The model under review builds one solid part; all positions refer to its coordinate system, in mm. Face numbers are marked on the shaded views. A direction names the side the tool comes from. Coordinates: 2 decimals unless noted, no trailing zeros. Loops run counter-clockwise (first coordinate to the right, second up) from the corner with the lowest first, then second, coordinate; pieces in that order, holes last. Notation, with made-up numbers: M 41,25 L 78,25 A12 cw 78,43 Z; hole C 9,25.25 d9. An arc over 180 degrees is marked long. Use one line per item in the form item = value.
```python
from build123d import *

# Parameters (mm, degrees)
DODANIE_WYCI_GNI_CIE1_DEPTH       = 25
DODANIE_WYCI_GNI_CIE2_DEPTH       = 5
WYCI_GNI_CIE_CIENKA_CIANKA1_DEPTH = 70
ZAOKR_GLENIE1_R                   = 10


with BuildPart() as part:
    # Szkic1 → Dodanie-wyci_gni_cie1 (new body)
    with BuildSketch(Plane.XY):
        with BuildLine():
            Line((0, 15), (0, 20))
            ThreePointArc((0, 20), (-20, 0), (0, -20))
            Line((0, -20), (0, -15))
            ThreePointArc((0, -15), (-15, 0), (0, 15))
        make_face()
    extrude(amount=DODANIE_WYCI_GNI_CIE1_DEPTH)

    # Szkic2 → Dodanie-wyci_gni_cie2 (add)
    with BuildSketch(Plane.XY):
        with BuildLine():
            Line((0, 20), (0, 72))
            Line((0, 72), (-40, 72))
            Line((-40, 72), (-40, 50.70936694))
            ThreePointArc((-40, 50.70936694), (-58.888387013, -17.302808514), (0, -56.220478651))
            Line((0, -56.220478651), (0, -20))
            Line((0, -20), (0, -15))
            ThreePointArc((0, -15), (-15, 0), (0, 15))
            Line((0, 15), (0, 20))
        make_face()
    extrude(amount=DODANIE_WYCI_GNI_CIE2_DEPTH)


with BuildPart() as body_2:
    # Lustro4: mirrored copy
    add(part.part.mirror(Plane(origin=(0, 0, -35), x_dir=(1, 0, 0), z_dir=(0, 0, -1))))


with BuildPart() as part_1:
    add(part.part)

    add(body_2.part)  # Wyci_gni_cie-cienka _cianka1 merges body 2
    # Szkic14 → Wyci_gni_cie-cienka _cianka1 (add)
    with BuildSketch(Plane(origin=(0, 0, 0), x_dir=(-1, 0, 0), z_dir=(0, 0, -1))):
        with BuildLine():
            Line((40, 72), (40, 50.70936694))
            ThreePointArc((40, 50.70936694), (58.888387013, -17.302808514), (0, -56.220478651))
            Line((0, -56.220478651), (0.224300204, -51.225512243))
            ThreePointArc((0.224300204, -51.225512243), (54.609267077, -14.434561812), (35, 48.229425454))
            Line((35, 48.229425454), (35, 72))
            Line((35, 72), (40, 72))
        make_face()
    extrude(amount=WYCI_GNI_CIE_CIENKA_CIANKA1_DEPTH)

    # Zaokr_glenie1
    zaokr_glenie1_edges = [part_1.edges().sort_by_distance(p)[0] for p in [
        (-40, 61.35468347, 5),
        (-40, 61.35468347, -75),
    ]]
    fillet(zaokr_glenie1_edges, radius=ZAOKR_GLENIE1_R)


solid = part_1.part
```
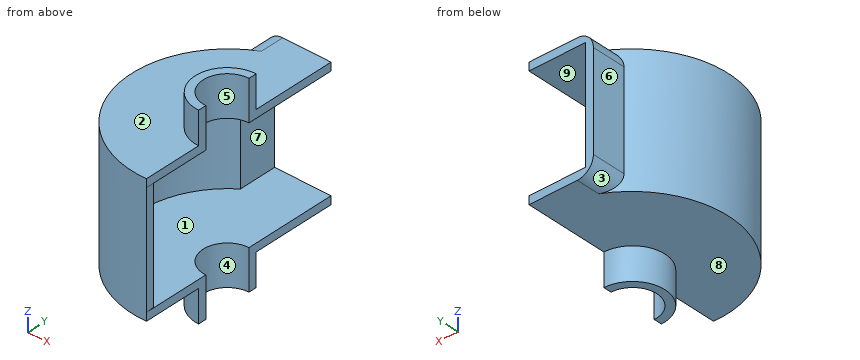
1. The part is to be moulded in two halves that separate along Z. For the marked faces 1, 2, 3 and 4, say which applies: pulls with the +Z half, pulls with the -Z half, needs draft (parallel to the pull), parting line crosses it, or undercut.
Response values:
face_1 = undercut
face_2 = pulls with the +Z half
face_3 = pulls with the -Z half
face_4 = needs draft
2. Add section B-B (x = -46.5). State the section outline as (y, z) points.
Response values:
outline = M -37.28,-75 L 44.72,-75 L 44.72,5 L -37.28,5 Z; hole M -29.53,-70 L 36.97,-70 L 36.97,0 L -29.53,0 Z
3. Wall thickness on line 1 along Z through (x, y) = (-35, 35); line 2 along Y through (x, z) = (-3.5, 19); line 3 along Z through (x, y) = (-50.5, -25.5): over which ranges is each line inside the solid? List them lowest first. Write a range as from..to.
Response values:
line_1 = -75..-70, 0..5
line_2 = -19.69..-14.59, 14.59..19.69
line_3 = -75..5
4. Machinability: for the marked faces 5, 6, 7, 8 and 9, which of the approach directions +Z, -Z, +X, -X, +Y, -Y give a long, thin tool a straight path to every point of the face, cutting with its end or side? Answer none if there is none.
Response values:
face_5 = +Z, -Z, +X
face_6 = +Z, -Z, -X, +Y
face_7 = +X, +Y
face_8 = -Z, -X
face_9 = +X
5. Add section C-C (z = -40). State the section outline as (x, y) points, then the cut area to 3 significant figures.
Response values:
outline = M -40,50.71 A60 ccw 0,-56.22 L -0.22,-51.23 A55 cw -35,48.23 L -35,72 L -40,72 Z
area = 842 mm^2
6. Add section D-D (x = -26). State the section outline as (y, z) points.
Response values:
outline = M -51.57,-75 L 72,-75 L 72,-70 L -46.1,-70 L -46.1,0 L 72,0 L 72,5 L -51.57,5 Z
7. Add section A-A (y = 59.5). State the section outline as (x, z) points, then the cut area to 3 significant figures.
Response values:
outline = M -40,-65 A10 ccw -30,-75 L 0,-75 L 0,-70 L -35,-70 L -35,0 L 0,0 L 0,5 L -30,5 A10 ccw -40,-5 Z
area = 707 mm^2
8. Insertion check: P1, Ø3, axis at y = 58, z = -59, coming from the +X side; P2, Ø3, axis at x = -35, y = 1, coming from the +Z side; P3, Ø12, axis at x = -41, z = -78, coming from the -Y side; P4, Ø10, axis at y = -40.5, z = -81, coming from the -X side. Each pin has a flat end and moves straight along its axis. Give the tip position at first contact, or say it passes through.
Response values:
P1 = -35
P2 = 5
P3 = -46.32
P4 = through
